from build123d import *

# Parameters (mm, degrees)
SKETCH1_R           = 3.5
SKETCH1_R_2         = 1
BOSS_EXTRUDE1_DEPTH = 3
SKETCH2_R           = 1
BOSS_EXTRUDE2_DEPTH = 2.5


with BuildPart() as part:
    # Sketch1 → Boss-Extrude1 (new body)
    with BuildSketch(Plane(origin=(0, 0, 0), x_dir=(1, 0, 0), z_dir=(0, 1, 0))):
        with BuildLine():
            Line((0, 18.516950365), (120, 9.258475183))
            ThreePointArc((120, 9.258475183), (129.258475183, 0), (120, -9.258475183))
            Line((120, -9.258475183), (0, -18.516950365))
            ThreePointArc((0, -18.516950365), (-18.516950365, 0), (0, 18.516950365))
        make_face()
        with Locations(Location((0, 0, 0), (0, 0, 270))):
            Circle(SKETCH1_R, mode=Mode.SUBTRACT)
        with Locations(Location((14.45, 0, 0), (0, 0, 270))):
            Circle(SKETCH1_R_2, mode=Mode.SUBTRACT)
        with Locations(Location((10.45, 0, 0), (0, 0, 270))):
            Circle(SKETCH1_R_2, mode=Mode.SUBTRACT)
    extrude(amount=BOSS_EXTRUDE1_DEPTH)

    # Sketch2 → Boss-Extrude2 (add)
    with BuildSketch(Plane(origin=(0, 3, 0), x_dir=(1, 0, 0), z_dir=(0, 1, 0))):
        with Locations(Location((-16, 0, 0), (0, 0, 270))):
            Circle(SKETCH2_R)
        with Locations(Location((0, 16, 0), (0, 0, 270))):
            Circle(SKETCH2_R)
        with Locations(Location((0, -16, 0), (0, 0, 270))):
            Circle(SKETCH2_R)
        with Locations(Location((127.5, 0, 0), (0, 0, 270))):
            Circle(SKETCH2_R)
    extrude(amount=BOSS_EXTRUDE2_DEPTH)


solid = part.part
Verification items for the finished model (mm, model axes). Give positions to 0.01 mm unless a question says otherwise; leave off trailing zeros. Loops run counter-clockwise (first coordinate to the right, second up) from the corner with the lowest first, then second, coordinate; pieces in that order, holes last. Notation, with made-up numbers: (25.25, -33) - (69.25, -33) arc R15 cw to (69.25, -10) - close; hole circle Ø2 at (23.5, -35). An arc over 180 degrees is marked (long way). Write item = value, one per line. Start each with the question number.
Q1. Cross-section at C-C, the plane z = -5. Enter the section's corners in (x, y), and give its area (3 significant figures).
Q2. Mould release check, pull along Z, two halves, no side actions. Record for faces 1 (the face through (129.256, 1.479, -0.204)), 2 (the face through (60.84, 1.479, 13.823)), 3 (the face through (-3.417, 1.479, -0.759)), 4 (the face through (56, 0, 0)): released by +Z, released by -Z, zero draft, split by the parting line, or undercut.
Q3. Depth check by flat-ended pin: P1, Ø8, axis at x = 98.5, z = -4.5, coming from the +Y side; P2, Ø1, axis at x = 43.5, y = 0.5, coming from the -Z side. Enter the tip coordinate at first touch or a pass-through.
Q4. Cross-section at A-A, the plane y = 1.05. Enter the section's corners in (x, z).
Q5. Thickness scan on line 1 (X direction, y = 2.1, z = 0); line 2 (Y direction, x = -9, z = -2.5); line 3 (X direction, y = 3.45, z = 0). Record the ranges inside material, lowest first.
Q6. Cross-section at B-B, the plane x = 109. Enter the section's corners in (y, z), and give its area (3 significant figures).
Answer key:
q1.outline = (-17.83, 0) - (127.79, 0) - (127.79, 3) - (-17.83, 3) - close
q1.area = 437 mm^2
q2.face_1 = split by the parting line
q2.face_2 = released by +Z
q2.face_3 = undercut
q2.face_4 = zero draft
q3.P1 = 3
q3.P2 = -15.2
q4.outline = (0, -18.52) - (120, -9.26) arc R9.26 ccw to (120, 9.26) - (0, 18.52) arc R18.52 ccw to start; hole circle Ø7 at (0, 0); hole circle Ø2 at (10.45, 0); hole circle Ø2 at (14.45, 0)
q5.line_1 = -18.52 to -3.5, 3.5 to 9.45, 11.45 to 13.45, 15.45 to 129.26
q5.line_2 = 0 to 3
q5.line_3 = -17 to -15, 126.5 to 128.5
q6.outline = (0, -10.11) - (3, -10.11) - (3, 10.11) - (0, 10.11) - close
q6.area = 60.6 mm^2
